Input: part model. Units: mm. Frame: model coordinates. Face numbers are marked on the shaded views. Coordinates: 2 decimals unless noted, no trailing zeros. Loops run counter-clockwise (first coordinate to the right, second up) from the corner with the lowest first, then second, coordinate; pieces in that order, holes last. Notation, with made-up numbers: (58, 71.25) - (109, 71.25) arc R24 cw to (109, 88.25) - close; hole circle Ø7 at (38, -1). An arc over 180 degrees is marked (long way). Use a Markdown table: item, result. Add a question column.
1. Section query C-C on x = -11. Return the cut outline in (y, z), then the cut area to 3 significant figures.
2. Section query A-A on y = -180.5. Return the cut outline in (x, z) (3 decimals), then the cut area to 3 significant figures.
3. Draft query along X for the marked faces 1, 2 and 3. Return one class per face: released by +X, released by -X, zero draft, split by the parting line, or undercut.
4. Ray query, L1, parallel to Z at x = 4, y = -105; L2, parallel to Z at x = 3, y = -174.5; L3, parallel to X at y = -24, z = -4. Return the intervals inside material, ascending. Write a range as [from, to].
5. Section query D-D on z = 9. Return the cut outline in (x, y), then the cut area to 3 significant figures.
6. Contact query for flat-ended pins moving along their axis: P1, Ø4, axis at x = 17.5, y = -90, coming from the -Z side; P2, Ø1, axis at x = 16.5, y = -117.5, coming from the +Z side; P3, Ø3, axis at x = 17.5, y = -149.5, coming from the -Z side. Output: stop coordinate, or through.
7. Section query B-B on z = -3. Return the cut outline in (x, y).
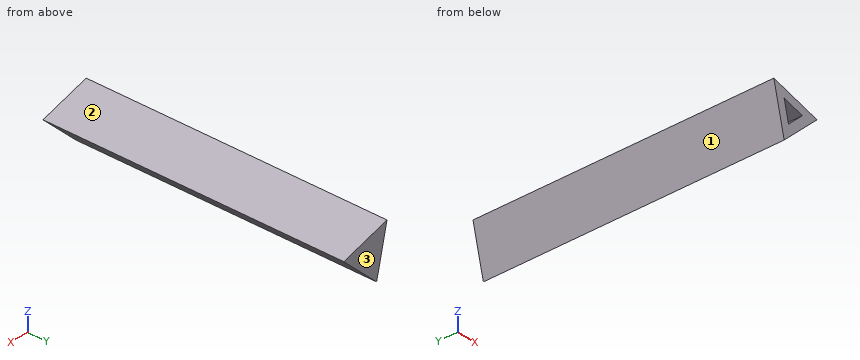
```python
from build123d import *

# Parameters (mm, degrees)
F1_DEPTH = 228.6
F2_T     = -6.35


with BuildPart() as f1:
    # F0 (on Front) → F1 (new body)
    with BuildSketch(Plane.XZ):
        Polygon((21.407872, 5.056975), (-15.083405, 16.011274), (-6.324467, -21.068249), align=None)
    extrude(amount=F1_DEPTH)

    # F2
    f2_openings = [f1.faces().sort_by_distance(p)[0] for p in [
        (0, -228.6, 0),
    ]]
    offset(amount=F2_T, openings=f2_openings)


solid = f1.part
```
Resolved:
| question | item | result |
|---|---|---|
| 1 | outline | (-228.6, -1.28) - (0, -1.28) - (0, 14.79) - (-228.6, 14.79) - close |
| 1 | area | 3,670 mm² |
| 2 | outline | (-15.083, 16.011) - (-6.324, -21.068) - (21.408, 5.057) - close; hole (-6.375, 6.767) - (-2.673, -8.904) - (9.048, 2.137) - close |
| 2 | area | 516 mm² |
| 3 | face 1 | released by -X |
| 3 | face 2 | released by +X |
| 3 | face 3 | zero draft |
| 4 | L1 | [-11.34, -2.62], [3.65, 10.28] |
| 4 | L2 | [-12.28, -3.56], [3.95, 10.58] |
| 4 | L3 | [-10.36, -3.83], [2.53, 11.79] |
| 5 | outline | (-13.43, -228.6) - (8.27, -228.6) - (8.27, 0) - (-13.43, 0) - close |
| 5 | area | 4,960 mm² |
| 6 | P1 | z = -0.51 |
| 6 | P2 | z = 6.68 |
| 6 | P3 | z = -0.04 |
| 7 | outline | (-10.59, -228.6) - (-4.07, -228.6) - (-4.07, -6.35) - (3.59, -6.35) - (3.59, -228.6) - (12.86, -228.6) - (12.86, 0) - (-10.59, 0) - close |
